Here's how the part is built. I have some questions about the finished solid (model axes, mm). Face numbers are marked on the shaded views. A direction names the side the tool comes from. Round coordinates to 2 decimals unless told otherwise and drop trailing zeros. Write each loop counter-clockwise with the first axis right and the second up, starting at its lowest first coordinate (ties: lowest second). Pieces come first, ordered by that corner, then holes. Notation, with made-up numbers: (51.5, 69.5) -> (108.5, 69.5) arc R10 cw to (108.5, 74.5) -> close; hole circle Ø4 at (-24, -23.5). An arc over 180 degrees is marked (long way). Answer in a Markdown table with one row per item.
Autodesk Inventor part; units mm, degrees
ref_plane "YZ Plane" through (0, 0, 0) normal (1, 0, 0) x (0, 1, 0)
ref_plane "XZ Plane" through (0, 0, 0) normal (0, 1, 0) x (-1, 0, 0)
ref_plane "XY Plane" through (0, 0, 0) normal (0, 0, 1) x (1, 0, 0)
sketch "servo_base" plane through (0, 0, 0) normal (0, 1, 0) x (-1, 0, 0)
  line L0 (-9.9, 10) -> (9.9, 10)
  line L1 (9.9, 10) -> (9.9, -30.6)
  line L2 (9.9, -30.6) -> (-9.9, -30.6)
  line L3 (-9.9, -30.6) -> (-9.9, 10)
  point P0 (0, 0)
  dimension "length" = 40.6
  dimension "width" = 19.8
  dimension "axe_dist" = 10
  dimension "d3" = 9.9
extrude "servo_body" add sketch "servo_base" along normal blind 36.6
sketch "handle1_base" plane through (-9.9, 0, 10) normal (0, 0, 1) x (1, 0, 0)
  line L0 (19.8, 0) -> (0, 0)
  line L1 (19.8, 0) -> (19.8, 36.6)
  line L2 (0, 0) -> (0, 36.6)
  line L3 (0, 26.8) -> (19.8, 26.8)
  line L4 (19.8, 26.8) -> (19.8, 29.8)
  line L5 (19.8, 29.8) -> (0, 29.8)
  line L6 (0, 29.8) -> (0, 26.8)
  point P0 (9.9, 0)
  dimension "handle_height" = 26.8
  dimension "handle_thickness" = 3
extrude "handle1" add sketch "handle1_base" along normal blind 6.4 contours L3 L2 L5 L1
sketch "handle2_base" plane through (9.9, 0, -30.6) normal (0, 0, -1) x (-1, 0, 0)
  line L0 (19.8, 0) -> (0, 0)
  line L1 (19.8, 0) -> (19.8, 36.6)
  line L2 (0, 0) -> (0, 36.6)
  line L3 (0, 26.8) -> (19.8, 26.8)
  line L4 (19.8, 26.8) -> (19.8, 29.8)
  line L5 (19.8, 29.8) -> (0, 29.8)
  line L6 (0, 29.8) -> (0, 26.8)
  point P0 (9.9, 0)
  dimension "d10" = 26.8
  dimension "d11" = 3
extrude "handle2" add sketch "handle2_base" along normal blind 6.4 contours L3 L2 L5 L1
sketch "hole1_right_base" plane through (-9.9, 29.8, 10) normal (0, 1, 0) x (1, 0, 0)
  line L0 (19.8, -6.4) -> (0, -6.4)
  line L1 (19.8, 0) -> (19.8, -6.4)
  line L2 (0, 0) -> (9.9, 0)
  line L3 (9.9, 0) -> (9.9, -6.4)
  line L4 (9.9, -6.4) -> (0, -6.4)
  line L5 (0, -6.4) -> (0, 0)
  circle A0 centre (4.9, -3.2) radius 2.5
  point P0 (9.9, 10)
  dimension "d14" = 9.9
  dimension "hole_dist" = 5
  dimension "d16" = 3.2
  dimension "hole_diameter" = 5
extrude "hole1_rigth" cut sketch "hole1_right_base" against normal up to next contours A0
sketch "hole1_left_base" plane through (-9.9, 29.8, 10) normal (0, 1, 0) x (1, 0, 0)
  line L0 (0, 0) -> (0, -6.4)
  line L1 (19.8, -6.4) -> (0, -6.4)
  line L2 (19.8, 0) -> (9.9, 0)
  line L3 (9.9, 0) -> (9.9, -6.4)
  line L4 (9.9, -6.4) -> (19.8, -6.4)
  line L5 (19.8, -6.4) -> (19.8, 0)
  circle A0 centre (14.9, -3.2) radius 2.5
  point P0 (9.9, 10)
  dimension "d20" = 9.9
  dimension "d21" = 3.2
  dimension "d22" = 5
  dimension "d23" = 5
extrude "hole1_left" cut sketch "hole1_left_base" against normal up to next contours A0
sketch "hole2_right_base" plane through (-9.9, 29.8, -30.6) normal (0, 1, 0) x (1, 0, 0)
  line L0 (19.8, 0) -> (0, 0)
  line L1 (19.8, 0) -> (19.8, 6.4)
  line L2 (0, 6.4) -> (19.8, 6.4)
  line L3 (0, 6.4) -> (9.9, 6.4)
  line L4 (9.9, 6.4) -> (9.9, 0)
  line L5 (9.9, 0) -> (0, 0)
  line L6 (0, 0) -> (0, 6.4)
  circle A0 centre (4.9, 3.2) radius 2.5
  point P0 (9.9, -30.6)
  dimension "d26" = 9.9
  dimension "d27" = 5
  dimension "d28" = 3.2
  dimension "d29" = 5
extrude "hole2_right" cut sketch "hole2_right_base" against normal up to next contours A0
sketch "hole2_left_base" plane through (-9.9, 29.8, -30.6) normal (0, 1, 0) x (1, 0, 0)
  line L0 (19.8, 0) -> (0, 0)
  line L1 (0, 6.4) -> (19.8, 6.4)
  line L2 (0, 0) -> (0, 6.4)
  line L3 (19.8, 6.4) -> (9.9, 6.4)
  line L4 (9.9, 6.4) -> (9.9, 0)
  line L5 (9.9, 0) -> (19.8, 0)
  line L6 (19.8, 0) -> (19.8, 6.4)
  circle A0 centre (14.9, 3.2) radius 2.5
  point P0 (9.9, -30.6)
  dimension "d32" = 9.9
  dimension "d33" = 5
  dimension "d34" = 5
  dimension "d35" = 3.2
extrude "hole2_left" cut sketch "hole2_left_base" against normal up to next contours A0
sketch "axe_base" plane through (0, 36.6, 0) normal (0, 1, 0) x (1, 0, 0)
  circle A0 centre (0, 0) radius 3
  line L0 (-9.9, -10) -> (9.9, -10)
  line L1 (0, 0) -> (0, -10) construction
  dimension "axe_diameter" = 6
  dimension "d41" = 10
extrude "axe" add sketch "axe_base" along normal blind 6.7
equation "\"d10\" = handle_height"
equation "\"d11\" = handle_thickness"
equation "\"d12\" = handle_length"
equation "\"d14\" = 0.5 * width"
equation "\"d16\" = 0.5 * handle_length"
equation "\"d18\" = handle_length"
equation "\"d20\" = 0.5 * width"
equation "\"d21\" = 0.5 * handle_length"
equation "\"d22\" = hole_dist"
equation "\"d23\" = hole_diameter"
equation "\"d24\" = handle_length"
equation "\"d26\" = 0.5 * width"
equation "\"d27\" = hole_dist"
equation "\"d28\" = 0.5 * handle_length"
equation "\"d29\" = hole_diameter"
equation "\"d30\" = handle_length"
equation "\"d32\" = 0.5 * width"
equation "\"d33\" = hole_diameter"
equation "\"d34\" = hole_dist"
equation "\"d35\" = 0.5 * handle_length"
equation "\"d36\" = handle_length"
properties part number "servo"
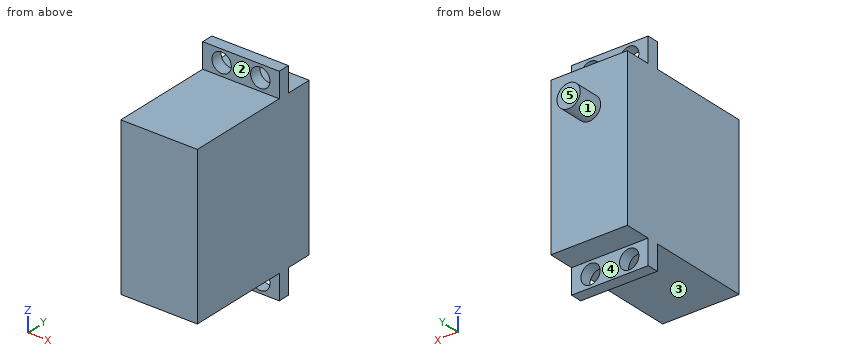
1) I need wall thicknesses on line 1 (Z direction, x = -5, y = 29.2); line 2 (X direction, y = 27, z = 13); line 3 (Z direction, x = 2, y = 13). Which ranges of each line are inside material? Lowest first, please. Write a range as [from, to].
Response:
| item | result |
|---|---|
| line 1 | z = [-37, -36.3], [-31.3, 10.7], [15.7, 16.4] |
| line 2 | x = [-9.9, -7.49], [-2.51, 2.51], [7.49, 9.9] |
| line 3 | z = [-30.6, 10] |
2) I want a section at B-B, the plane y = 28. List the corners of the cut face in (x, z) for me.
Response:
| item | result |
|---|---|
| outline | (-9.9, -37) -> (9.9, -37) -> (9.9, 16.4) -> (-9.9, 16.4) -> close; hole circle Ø5 at (-5, -33.8); hole circle Ø5 at (-5, 13.2); hole circle Ø5 at (5, -33.8); hole circle Ø5 at (5, 13.2) |
3) I want a section at A-A, the plane x = -5. List the corners of the cut face in (y, z) for me.
Response:
| item | result |
|---|---|
| outline | (0, -30.6) -> (26.8, -30.6) -> (26.8, -31.3) -> (29.8, -31.3) -> (29.8, -30.6) -> (36.6, -30.6) -> (36.6, 10) -> (29.8, 10) -> (29.8, 10.7) -> (26.8, 10.7) -> (26.8, 10) -> (0, 10) -> close; (26.8, -37) -> (29.8, -37) -> (29.8, -36.3) -> (26.8, -36.3) -> close; (26.8, 15.7) -> (29.8, 15.7) -> (29.8, 16.4) -> (26.8, 16.4) -> close |
4) For pin 1 (10 mm diameter, centred on x = -0.5, y = 8, fed in from +Z); pin 2 (4 mm diameter, centred on x = 6.5, z = -30, fed in from +Y); pin 3 (6 mm diameter, centred on x = -5, z = -33.8, fed in from +Y), each with a flat end and sliding along its axis, tell me the tip position at first contact or that it passes through.
Response:
| item | result |
|---|---|
| pin 1 | stops at z = 10 |
| pin 2 | stops at y = 36.6 |
| pin 3 | stops at y = 29.8 |
5) Which directions (+Z, -Z, +X, -X, +Y, -Y) give clear straight access to the entire face, cutting with the end or side of a thin tool? Please do the marked faces 1, 2, 3, 4 and 5.
Response:
| item | result |
|---|---|
| face 1 | +Y |
| face 2 | +Z, +X, -X, -Y |
| face 3 | -Z, +X, -X, -Y |
| face 4 | -Z, +X, -X, +Y |
| face 5 | +Z, -Z, +X, -X, +Y |
6) I want a section at C-C, the plane z = -33.8. List the corners of the cut face in (x, y) for me, and give its area (3 significant figures).
Response:
| item | result |
|---|---|
| outline | (-9.9, 26.8) -> (-7.5, 26.8) -> (-7.5, 29.8) -> (-9.9, 29.8) -> close; (-2.5, 26.8) -> (2.5, 26.8) -> (2.5, 29.8) -> (-2.5, 29.8) -> close; (7.5, 26.8) -> (9.9, 26.8) -> (9.9, 29.8) -> (7.5, 29.8) -> close |
| area | 29.4 mm^2 |
7) I want a section at D-D, the plane x = 0. List the corners of the cut face in (y, z) for me, and give its area (3 significant figures).
Response:
| item | result |
|---|---|
| outline | (0, -30.6) -> (26.8, -30.6) -> (26.8, -37) -> (29.8, -37) -> (29.8, -30.6) -> (36.6, -30.6) -> (36.6, -3) -> (43.3, -3) -> (43.3, 3) -> (36.6, 3) -> (36.6, 10) -> (29.8, 10) -> (29.8, 16.4) -> (26.8, 16.4) -> (26.8, 10) -> (0, 10) -> close |
| area | 1,560 mm^2 |
